Geometry: final body of the model. Coordinates: model frame, mm. A direction names the side the tool comes from. Give positions to 0.01 mm unless a question says otherwise; leave off trailing zeros. Write each loop counter-clockwise with the first axis right and the second up, starting at its lowest first coordinate (ties: lowest second). Pieces come first, ordered by that corner, then holes.
Autodesk Inventor part; units mm, degrees
ref_plane "YZ Plane" through (0, 0, 0) normal (1, 0, 0) x (0, 1, 0)
ref_plane "XZ Plane" through (0, 0, 0) normal (0, 1, 0) x (-1, 0, 0)
ref_plane "XY Plane" through (0, 0, 0) normal (0, 0, 1) x (1, 0, 0)
sketch "Sketch1" plane through (0, 0, 0) normal (0, 1, 0) x (-1, 0, 0)
  line L0 (-13, 13) -> (13, 13)
  line L1 (13, 13) -> (13, -13)
  line L2 (13, -13) -> (-13, -13)
  line L3 (-13, -13) -> (-13, 13)
  line L4 (-13, 13) -> (13, -13) construction
  line L5 (13, 13) -> (-13, -13) construction
  circle A0 centre (11.5, 11.5) radius 1
  line L6 (0, 0) -> (3.4228, 0) construction
  line L7 (0, 0) -> (0, 5.3357) construction
  circle A1 centre (11.5, -11.5) radius 1
  circle A2 centre (-11.5, 11.5) radius 1
  circle A3 centre (-11.5, -11.5) radius 1
  dimension "d0" = 26
  dimension "d1" = 26
  dimension "d2" = 2
  dimension "d3" = 1.5
extrude "Extrusion1" add sketch "Sketch1" along normal blind 1
sketch "Sketch2" plane through (0, 1, 0) normal (0, 1, 0) x (1, 0, 0)
  line L0 (-13, 13) -> (-13, -13) construction
  line L1 (0, 0) -> (-10.4427, 0) construction
  line L2 (7.5, -12.5) -> (-9, -12.5)
  line L3 (-9, -12.5) -> (-9, 12.5)
  line L4 (-9, 12.5) -> (7.5, 12.5)
  line L5 (7.5, 12.5) -> (7.5, -12.5)
  line L6 (7.5, -12.5) -> (-9, 12.5) construction
  line L7 (-9, -12.5) -> (7.5, 12.5) construction
  point P0 (-0.75, 0)
  dimension "d6" = 16.5
  dimension "d7" = 25
  dimension "d8" = 4
extrude "Extrusion2" add sketch "Sketch2" along normal blind 1.5
properties part number "Screen"
Q1. Ray query, line 1 along Z through (x, y) = (11.5, 0.6); line 2 along Z through (x, y) = (4.75, 1.25); line 3 along X through (y, z) = (1.7, -7.25). Return the intervals inside material, ascending.
Filled sheet:
line 1: z = -13 to -12.5, -10.5 to 10.5, 12.5 to 13
line 2: z = -12.5 to 12.5
line 3: x = -9 to 7.5
Q2. Section B-B on z = -11.5. Output: boundary loops of the cut face in (x, y).
Filled sheet:
outline: (-13, 0) - (-12.5, 0) - (-12.5, 1) - (-13, 1) - close; (-10.5, 0) - (10.5, 0) - (10.5, 1) - (7.5, 1) - (7.5, 2.5) - (-9, 2.5) - (-9, 1) - (-10.5, 1) - close; (12.5, 0) - (13, 0) - (13, 1) - (12.5, 1) - close
Q3. Pin query (flat end, axial travel): P1, Ø2.5, axis at x = 11.5, z = 11.5, coming from the +Y side; P2, Ø0.8, axis at y = 1.5, z = 6, coming from the +X side. Return the tip coordinate at first contact, or that it passes through.
Filled sheet:
P1: stops at y = 1
P2: stops at x = 7.5
Q4. Section D-D on x = -3.5. Output: boundary loops of the cut face in (y, z), plus the area to 3 significant figures.
Filled sheet:
outline: (0, -13) - (1, -13) - (1, -12.5) - (2.5, -12.5) - (2.5, 12.5) - (1, 12.5) - (1, 13) - (0, 13) - close
area: 63.5 mm2
Q5. Pull-direction query (Z, two-part tool) for faces 1 (the flat face through (7.5, 2, 0)), 2 (the cylindrical face through (-10.763, 0.493, 10.824)), 3 (the flat face through (-0.2, 0.5, -13)); classes: released by +Z, released by -Z, zero draft, split by the parting line, or undercut.
Filled sheet:
face 1: zero draft
face 2: undercut
face 3: released by -Z
Q6. Section A-A on x = 11.5. Output: boundary loops of the cut face in (y, z).
Filled sheet:
outline: (0, -13) - (1, -13) - (1, -12.5) - (0, -12.5) - close; (0, -10.5) - (1, -10.5) - (1, 10.5) - (0, 10.5) - close; (0, 12.5) - (1, 12.5) - (1, 13) - (0, 13) - close
Q7. Access query for faces 4 (the flat face through (0.2, 0.5, 13)), 5 (the flat face through (-1, 2, -12.5)), 6 (the flat face through (-1, 2, 12.5)), 7 (the flat face through (-9, 2, 0)), 8 (the flat face through (-1, 2.5, 0)). Directions: +Z, -Z, +X, -X, +Y, -Y. A direction counts if a zero-diameter tool reaches every point of the face in a straight line with its end or side. Return the directions, or none.
Filled sheet:
face 4: +Z, +X, -X, +Y, -Y
face 5: -Z, +X, -X, +Y
face 6: +Z, +X, -X, +Y
face 7: +Z, -Z, -X, +Y
face 8: +Z, -Z, +X, -X, +Y
Q8. Section C-C on y = 0.4. Output: boundary loops of the cut face in (x, z), plus the area to 3 significant figures.
Filled sheet:
outline: (-13, -13) - (13, -13) - (13, 13) - (-13, 13) - close; hole circle Ø2 at (-11.5, -11.5); hole circle Ø2 at (-11.5, 11.5); hole circle Ø2 at (11.5, -11.5); hole circle Ø2 at (11.5, 11.5)
area: 663 mm2
